Can you work these out from the model? Positions are in its coordinate system, mm. A direction names the side the tool comes from. Round coordinates to 2 decimals unless told otherwise and drop trailing zeros. Write each loop counter-clockwise with the first axis right and the second up, starting at its lowest first coordinate (ties: lowest second). Pieces come first, ordered by that corner, then holes. Notation, with made-up numbers: (-20, 44.25) -> (25, 44.25) arc R29 cw to (25, 79.25) -> close; hole circle Ø1 at (59, 39.25). An arc over 180 degrees is marked (long way). Write item = value, one per line. Start each with the question number.
1) For faces 1 (the face through (1, 91, -7)), 2 (the face through (0, 91, -6)), which set-ups out of +Z, -Z, +X, -X, +Y, -Y let a thin tool reach every point of the face, with its end or its side?
2) I'm going to push flat-ended pins straight in: pin 1 (7 mm diameter, centred on x = 6.5, y = 123, fed in from -Z); pin 2 (2 mm diameter, centred on x = 10, y = 176, fed in from -Z); pin 3 (3 mm diameter, centred on y = 177, z = -7, fed in from +X). Where does each tip first touch, or does it pass through?
3) Imagine slicing it at A-A, the plane y = 106.5. Please give me the cut outline in (x, z).
4) Imagine slicing it at B-B, the plane z = -11.75. Please give me the cut outline in (x, y).
5) If I drill on line 1 (Y direction, x = 0.75, z = -7); line 2 (Y direction, x = 10, z = 0.75); line 3 (X direction, y = 176, z = 0.2), over which ranges is the centre line in solid material (lowest first)?
6) Imagine slicing it at C-C, the plane x = 3. Please give me the cut outline in (y, z).
from build123d import *

# Parameters (mm, degrees)
SKETCH_1_W      = 15
SKETCH_1_H      = 1
EXTRUDE_1_DEPTH = 184
SKETCH_3_W      = 1
SKETCH_3_H      = 184
EXTRUDE_2_DEPTH = 14
M3X0_5_1_D      = 2.5
M3X0_5_2_D      = 2.5


with BuildPart() as part:
    # ｽｹｯﾁ1 → ﾎﾞｽ - 押し出し1 (new body)
    with BuildSketch(Plane(origin=(0, 0, 0), x_dir=(1, 0, 0), z_dir=(0, 1, 0))):
        with Locations((7.5, -0.5)):
            Rectangle(SKETCH_1_W, SKETCH_1_H)
    extrude(amount=EXTRUDE_1_DEPTH)

    # ｽｹｯﾁ3 → ﾎﾞｽ - 押し出し2 (add)
    with BuildSketch(Plane(origin=(0, 0, 0), x_dir=(-1, 0, 0), z_dir=(0, 0, -1))):
        with Locations((-0.5, 92)):
            Rectangle(SKETCH_3_W, SKETCH_3_H)
    extrude(amount=EXTRUDE_2_DEPTH)

    # M3x0.5 ねじ穴1 (through all)
    with Locations(Plane.ZY):
        with Locations((-7, 7), (-7, 177)):
            Hole(M3X0_5_1_D / 2)

    # M3x0.5 ねじ穴2 (through all)
    with Locations(Plane.XY.offset(1)):
        with Locations((10, 8), (10, 176)):
            Hole(M3X0_5_2_D / 2)


solid = part.part
Reported:
q1.face_1 = -Z, +X, +Y, -Y
q1.face_2 = +Z, -Z, -X, +Y, -Y
q2.pin_1 = 0
q2.pin_2 = through
q2.pin_3 = 1
q3.outline = (0, -14) -> (1, -14) -> (1, 0) -> (15, 0) -> (15, 1) -> (0, 1) -> close
q4.outline = (0, 0) -> (1, 0) -> (1, 184) -> (0, 184) -> close
q5.line_1 = 0 to 5.75, 8.25 to 175.75, 178.25 to 184
q5.line_2 = 0 to 6.75, 9.25 to 174.75, 177.25 to 184
q5.line_3 = 0 to 8.75, 11.25 to 15
q6.outline = (0, 0) -> (184, 0) -> (184, 1) -> (0, 1) -> close
